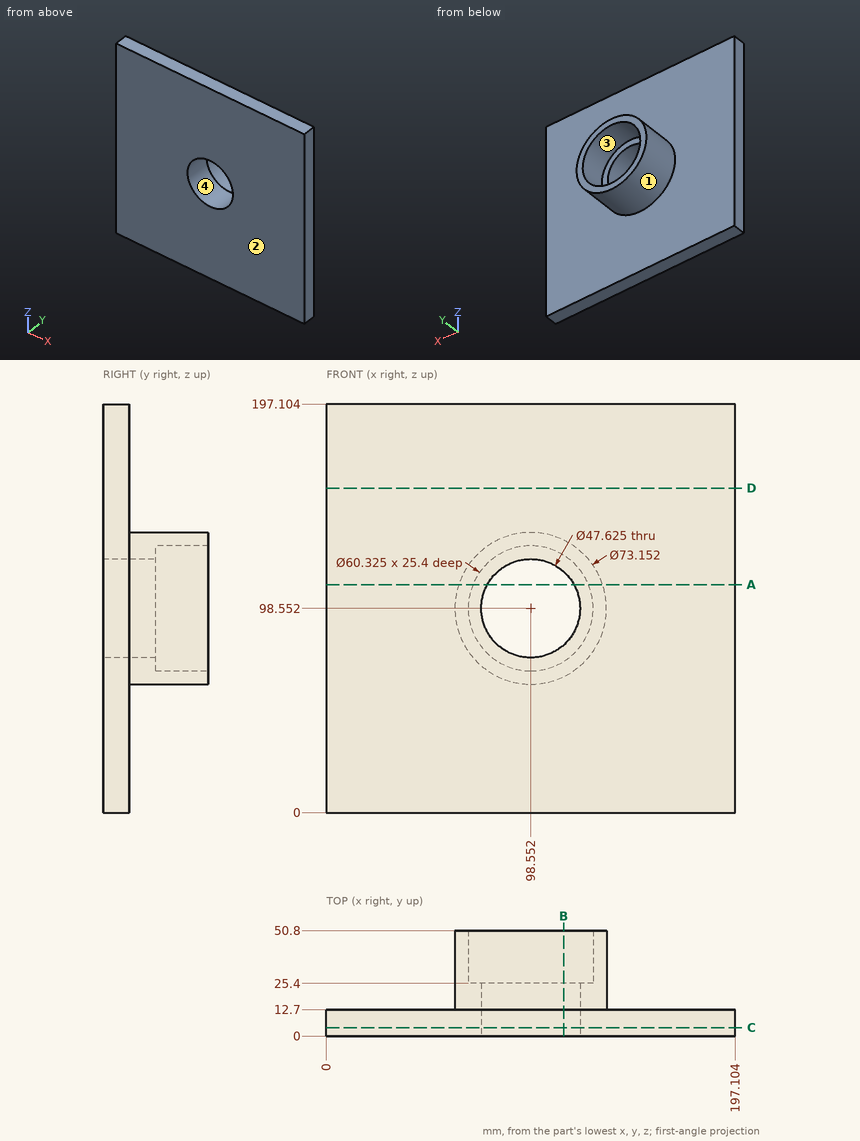
The drawing under review shows one solid part. Ordinate dimensions are in mm from its lowest x, y, z. Coordinates: 2 decimals unless noted, no trailing zeros. Write each loop counter-clockwise with the first axis right and the second up, starting at its lowest first coordinate (ties: lowest second). Pieces come first, ordered by that corner, then holes. Notation, with made-up numbers: (44, 26) - (85, 26) arc R22 ccw to (85, 63) - close; hole circle Ø5 at (-39.5, -36). An arc over 180 degrees is marked (long way). Put each result on its own line as item: value.
1. Wall thickness on probe 1 along X at (y, z) = (2.5, 100); probe 2 along Y at (x, z) = (146.5, 95.5); probe 3 along X at (y, z) = (33.5, 111): over which ranges is each line inside the solid? List them lowest first.
Values found:
probe 1: 0 to 74.78, 122.32 to 197.1
probe 2: 0 to 12.7
probe 3: 64.16 to 71.08, 126.03 to 132.94
2. Add section D-D, the plane z = 156.5. Give the boundary of the cut face in (x, y).
Values found:
outline: (0, 0) - (197.1, 0) - (197.1, 12.7) - (0, 12.7) - close
3. Add section B-B, the plane x = 114.5. Give the boundary of the cut face in (y, z).
Values found:
outline: (0, 0) - (12.7, 0) - (12.7, 65.64) - (50.8, 65.64) - (50.8, 72.95) - (25.4, 72.95) - (25.4, 80.87) - (0, 80.87) - close; (0, 116.24) - (25.4, 116.24) - (25.4, 124.15) - (50.8, 124.15) - (50.8, 131.47) - (12.7, 131.47) - (12.7, 197.1) - (0, 197.1) - close
4. Add section C-C, the plane y = 4. Give the boundary of the cut face in (x, z) (1 decimal), then the cut area to 3 significant figures.
Values found:
outline: (0, 0) - (197.1, 0) - (197.1, 197.1) - (0, 197.1) - close; hole circle Ø47.6 at (98.6, 98.6)
area: 37,100 mm²
5. For pin 1 (1 mm diameter, centred on y = 26, z = 122.5, fed in from +X); pin 2 (8 mm diameter, centred on x = 121.5, y = 41.5, fed in from -Z); pin 3 (1.5 mm diameter, centred on x = 137, z = 157.5, fed in from +Y), all flat-tipped, find the tip position at first contact; note any pin that passes through.
Values found:
pin 1: x = 126.62
pin 2: z = 67.27
pin 3: y = 12.7
6. Mouldability with a two-part tool opening along X and no side actions: class the marked faces 1, 2, 3 and 4 as released by +X, released by -X, zero draft, split by the parting line, or undercut.
Values found:
face 1: split by the parting line
face 2: zero draft
face 3: undercut
face 4: undercut
7. Add section A-A, the plane z = 110. Give the boundary of the cut face in (x, y).
Values found:
outline: (0, 0) - (77.67, 0) - (77.67, 25.4) - (70.65, 25.4) - (70.65, 50.8) - (63.81, 50.8) - (63.81, 12.7) - (0, 12.7) - close; (119.43, 0) - (197.1, 0) - (197.1, 12.7) - (133.29, 12.7) - (133.29, 50.8) - (126.46, 50.8) - (126.46, 25.4) - (119.43, 25.4) - close
